from build123d import *

# Parameters (mm, degrees)
ESQUISSE1_W      = 28
ESQUISSE1_H      = 60
EXTRUSION1_DEPTH = 4


with BuildPart() as part:
    # Esquisse1 → Extrusion1 (new body)
    with BuildSketch(Plane(origin=(0, 0, 0), x_dir=(1, 0, 0), z_dir=(0, 1, 0))):
        with BuildLine():
            Line((110, 0), (-110, 0))
            ThreePointArc((-110, 0), (-131.213203436, -8.786796564), (-140, -30))
            Line((-140, -30), (-140, -260))
            ThreePointArc((-140, -260), (-131.213203436, -281.213203436), (-110, -290))
            Line((-110, -290), (110, -290))
            ThreePointArc((110, -290), (131.213203436, -281.213203436), (140, -260))
            Line((140, -260), (140, -30))
            ThreePointArc((140, -30), (131.213203436, -8.786796564), (110, 0))
        make_face()
        with Locations((70, -145)):
            Rectangle(ESQUISSE1_W, ESQUISSE1_H, mode=Mode.SUBTRACT)
        with Locations((-70, -145)):
            Rectangle(ESQUISSE1_W, ESQUISSE1_H, mode=Mode.SUBTRACT)
    extrude(amount=EXTRUSION1_DEPTH)


solid = part.part
Model file for the job. Use its own axes, mm. Round coordinates to 2 decimals unless told otherwise and drop trailing zeros. Order: outer loops, then holes, each group sorted by start corner. A loop starts at its lowest first (then second) coordinate and runs counter-clockwise, first axis right, second up.
(1) Band-saw the part on C-C (y = 1.7). List the corners of the cut face in (x, z).
(2) Drill centre lines: line 1 (X direction, y = 2.3, z = 169); line 2 (Z direction, x = -62.5, y = 2.8); line 3 (Z direction, x = -127, y = 0.3). Where is each one in solid material? Low to high.
(3) Band-saw the part on A-A (z = 125). List the corners of the cut face in (x, y), then the cut area to 3 significant figures.
(4) Band-saw the part on B-B (x = -77.5). List the corners of the cut face in (y, z), then the cut area to 3 significant figures.
Verdict:
1. outline: (-140, 30) arc R30 ccw to (-110, 0) - (110, 0) arc R30 ccw to (140, 30) - (140, 260) arc R30 ccw to (110, 290) - (-110, 290) arc R30 ccw to (-140, 260) - close; hole (-84, 115) - (-56, 115) - (-56, 175) - (-84, 175) - close; hole (56, 115) - (84, 115) - (84, 175) - (56, 175) - close
2. line 1: x = -140 to -84, -56 to 56, 84 to 140
2. line 2: z = 0 to 115, 175 to 290
2. line 3: z = 5.28 to 284.72
3. outline: (-140, 0) - (-84, 0) - (-84, 4) - (-140, 4) - close; (-56, 0) - (56, 0) - (56, 4) - (-56, 4) - close; (84, 0) - (140, 0) - (140, 4) - (84, 4) - close
3. area: 896 mm2
4. outline: (0, 0) - (4, 0) - (4, 115) - (0, 115) - close; (0, 175) - (4, 175) - (4, 290) - (0, 290) - close
4. area: 920 mm2
